from build123d import *

# Parameters (mm, degrees)
F0_R     = 19.05
F0_R_2   = 4.7625
F0_R_3   = 6.096
F0_R_4   = 45.72
F1_DEPTH = 12.7


# Not quite as in the source:
# - ends of sketch curves that miss each other by under 0.0002 mm in the source are joined


with BuildPart() as f1:
    # F0 (on Front) → F1 (new body)
    with BuildSketch(Plane.XZ):
        with BuildLine():
            Line((37.0673326191, 65.1785315794), (24.1799304387, 133.8380140911))
            Line((24.1799304387, 133.8380140911), (-26.6200695613, 133.8380140911))
            Line((-26.6200695613, 133.8380140911), (-37.9125978196, 64.6905174884))
            Line((-37.9125978196, 64.6905174884), (-47.7326956793, 47.4230339812))
            add(Edge.make_bspline(
                [(-47.7326956793, 47.4230339812), (-51.0448461758, 29.0294404336), (-51.0448462531, 29.0294404776), (-64.9358999582, 17.1732288977)],
                knots=[0, 0, 0, 0, 34.7994388611, 34.7994388611, 34.7994388611, 34.7994388611], degree=3))
            Line((-64.9358999582, 17.1732288977), (-74.9799305502, -0.4880138996))
            Line((-74.9799305502, -0.4880138996), (-64.9359000035, -17.6262099378))
            add(Edge.make_bspline(
                [(-64.9359000035, -17.6262099378), (-50.6626559715, -29.6914131837), (-50.6626551721, -29.6914132451), (-47.3404022927, -47.649524558)],
                knots=[0, 0, 0, 0, 34.7994390827, 34.7994390827, 34.7994390827, 34.7994390827], degree=3))
            Line((-47.3404022927, -47.649524558), (-37.0673327313, -65.1785313884))
            Line((-37.0673327313, -65.1785313884), (-26.6200695613, -132.8619859089))
            Line((-26.6200695613, -132.8619859089), (24.1799304387, -132.8619859089))
            Line((24.1799304387, -132.8619859089), (37.9125978196, -64.6905174884))
            Line((37.9125978196, -64.6905174884), (47.7326956902, -47.4230338593))
            add(Edge.make_bspline(
                [(64.9358998918, -17.1732287319), (51.0448461867, -29.0294403117), (51.0448461867, -29.0294403117), (47.7326956902, -47.4230338593)],
                knots=[0, 0, 0, 0, 34.7994388611, 34.7994388611, 34.7994388611, 34.7994388611], degree=3))
            Line((64.9358998918, -17.1732287319), (74.9799304387, 0.4880140911))
            Line((74.9799304387, 0.4880140911), (64.9358998918, 17.6262101292))
            add(Edge.make_bspline(
                [(47.3404022927, 47.649524558), (50.662655861, 29.6914133741), (50.662655861, 29.6914133741), (64.9358998918, 17.6262101292)],
                knots=[0, 0, 0, 0, 34.7994388611, 34.7994388611, 34.7994388611, 34.7994388611], degree=3))
            Line((47.3404022927, 47.649524558), (37.0673326191, 65.1785315794))
        make_face()
        with Locations((-1.2200695613, -96.0319859089)):
            Circle(F0_R, mode=Mode.SUBTRACT)
        with Locations((-30.4998691349, -50.180102728)):
            Circle(F0_R_2, mode=Mode.SUBTRACT)
        with Locations((28.6262483892, -51.2720453093)):
            Circle(F0_R_3, mode=Mode.SUBTRACT)
        Circle(F0_R_4, mode=Mode.SUBTRACT)
        with Locations((58.7220974339, 0)):
            Circle(F0_R_2, mode=Mode.SUBTRACT)
        with Locations((-58.7227720341, 0.4880365509)):
            Circle(F0_R_3, mode=Mode.SUBTRACT)
        with Locations((-30.0641650228, 50.4423503469)):
            Circle(F0_R_2, mode=Mode.SUBTRACT)
        with Locations((-1.2200695613, 97.0080140911)):
            Circle(F0_R, mode=Mode.SUBTRACT)
        with Locations((28.1997188878, 51.5078691239)):
            Circle(F0_R_3, mode=Mode.SUBTRACT)
    extrude(amount=F1_DEPTH)


solid = f1.part
Build history of the part. All positions in model axes, mm. Coordinates: 2 decimals unless noted, no trailing zeros. Order: outer loops, then holes, each group sorted by start corner. A loop starts at its lowest first (then second) coordinate and runs counter-clockwise, first axis right, second up. Notation, with made-up numbers: M -34,-8.5 L 4,-8.5 A20 ccw 4,16.5 Z; hole C 24,-35 d6. An arc over 180 degrees is marked long. One line per question, with ' | ' between items. Start each with the question number.
Q1. Two-plate mould, pull along X, no slides. Class faces 1 (the face through (70.028, -6.261, 8.937)), 2 (the face through (-2, -6, -132.862)), 3 (the face through (23.71, -6.26, 55.63)): +X half, -X half, draft (parallel to the pull), parting line (faces both ways), or undercut.
Q2. Saw through at D-D (y = -6). Count the separate pieces of the cut face and the enclosed holes in it, then the cut area to 3 significant figures.
Q3. Probe L1, parallel to Z at x = 15.5, y = -6.5; L2, parallel to X at y = -0.25, z = 51; L3, parallel to Z at x = 4, y = -6. List the from-to ranges inside material, lowest first. Write a range as from..to.
Q4. Saw through at C-C (z = 80.5). List the corners of the cut face in (x, y).
Q5. Flat gauge pins, fed straight in: pin 1 Ø1 at (y, z) = (-8, 31.5) entering from -X; pin 2 Ø2 at (y, z) = (-5.5, 48.5) entering from +X. Where does each tip first touch, or does it go through?
Q6. Saw through at A-A (z = -101.5). List the corners of the cut face in (x, y), then the cut area to 3 significant figures.
Q7. Saw through at B-B (x = 0). List the corners of the cut face in (y, z).
Check values:
1) face 1: +X half | face 2: draft | face 3: undercut
2) separate pieces: 1 | enclosed holes: 9 | area: 13,400 mm2
3) L1: z = -132.86..-105.16, -86.9..-43.01, 43.01..87.88, 106.14..133.84 | L2: x = -45.7..-34.79, -25.33..22.12, 34.27..45.38 | L3: z = -132.86..-114.35, -77.71..-45.54, 45.54..78.69, 115.33..133.84
4) outline: M -35.33,-12.7 L -10.73,-12.7 L -10.73,0 L -35.33,0 Z; M 8.29,-12.7 L 34.19,-12.7 L 34.19,0 L 8.29,0 Z
5) pin 1: stops at x = -51.76 | pin 2: stops at x = 47.37
6) outline: M -31.46,-12.7 L -19.47,-12.7 L -19.47,0 L -31.46,0 Z; M 17.03,-12.7 L 30.5,-12.7 L 30.5,0 L 17.03,0 Z | area: 323 mm2
7) outline: M -12.7,-132.86 L 0,-132.86 L 0,-115.04 L -12.7,-115.04 Z; M -12.7,-77.02 L 0,-77.02 L 0,-45.72 L -12.7,-45.72 Z; M -12.7,45.72 L 0,45.72 L 0,78 L -12.7,78 Z; M -12.7,116.02 L 0,116.02 L 0,133.84 L -12.7,133.84 Z
